Part model, mm, in its own coordinate system. A direction names the side the tool comes from. Round coordinates to 2 decimals unless told otherwise and drop trailing zeros. Write each loop counter-clockwise with the first axis right and the second up, starting at its lowest first coordinate (ties: lowest second). Pieces come first, ordered by that corner, then holes.
1) Drill centre lines: L1, parallel to Y at x = -35, z = 78; L2, parallel to X at y = 42, z = 18; L3, parallel to Z at x = -72.5, y = 26. Where is each one in solid material? Low to high.
2) Pull direction Z, two halves, no side cores. Call faces 1 (the flat face through (-22.76, -3.7, 105.18)), 2 (the flat face through (-81, -3, 0)), 3 (the flat face through (-28, -62.49, 40)), 4 (the flat face through (-26.974, -5.309, 113.826)): +Z half, -Z half, draft (parallel to the pull), parting line (faces both ways), or undercut.
3) Saw through at C-C on x = -71.5. Write the cut outline in (y, z), and give its area (3 significant figures).
4) Flat gauge pins, fed straight in: pin 1 (2 mm diameter, centred on x = -67, y = -57, fed in from -Z); pin 2 (2 mm diameter, centred on y = -2, z = 126, fed in from +X); pin 3 (1.5 mm diameter, centred on x = -33, y = 11.5, fed in from +Z). Where does each tip first touch, or does it go through?
5) Saw through at D-D on z = 86.5. Write the cut outline in (x, y), and give its area (3 significant figures).
6) Saw through at A-A on y = -22. Write the cut outline in (x, z) (3 decimals), and give its area (3 significant figures).
7) Which spindle directions (+Z, -Z, +X, -X, +Y, -Y) get a long thin tool onto all of the face, cutting with end or side? Do faces 5 (the flat face through (-79.493, -5, 52)), 6 (the flat face through (-51, -3, 105)), 7 (the flat face through (51.551, -5, 14)). Say none if no direction does.
8) Saw through at B-B on x = 34. Write the cut outline in (y, z).
```python
from build123d import *

# Parameters (mm, degrees)
SKETCH3_W           = 150
SKETCH3_H           = 150
BOSS_EXTRUDE2_DEPTH = 150
CUT_EXTRUDE3_DEPTH  = 150
SKETCH8_W           = 131.044313332
SKETCH8_H           = 116.977993985
CUT_EXTRUDE7_DEPTH  = 105
SKETCH9_W           = 4.954866237
SKETCH9_H           = 116.977993985
CUT_EXTRUDE10_DEPTH = 3
SKETCH10_W          = 105.341543671
SKETCH10_H          = 5
CUT_EXTRUDE12_DEPTH = 3
SKETCH11_W          = 5
SKETCH11_H          = 121.977993985
CUT_EXTRUDE13_DEPTH = 3
SKETCH12_W          = 110.341543671
SKETCH12_H          = 5
CUT_EXTRUDE14_DEPTH = 3


with BuildPart() as part:
    # Sketch3 → Boss-Extrude2 (new body)
    with BuildSketch(Plane.XY):
        with Locations((-13.712644514, -4.259252527)):
            Rectangle(SKETCH3_W, SKETCH3_H)
    extrude(amount=BOSS_EXTRUDE2_DEPTH)

    # Sketch6 → Cut-Extrude3 (cut)
    with BuildSketch(Plane.XZ.offset(79.259252527)):
        Polygon((61.287355486, 22.975304178), (-62.11733168, 150), (61.287355486, 150), align=None)
    extrude(amount=-CUT_EXTRUDE3_DEPTH, mode=Mode.SUBTRACT)

    # Sketch8 → Cut-Extrude7 (cut)
    with BuildSketch(Plane(origin=(0, 0, 0), x_dir=(-1, 0, 0), z_dir=(0, 0, -1))):
        with Locations((13.971216561, -4.00068048)):
            Rectangle(SKETCH8_W, SKETCH8_H)
    extrude(amount=-CUT_EXTRUDE7_DEPTH, mode=Mode.SUBTRACT)

    # Sketch9 → Cut-Extrude10 (cut)
    with BuildSketch(Plane(origin=(43.01226643, 0, 41.786482925), x_dir=(0.696812609304925, 0, -0.71725322412218), z_dir=(0.71725322412218, 0, 0.696812609304925))):
        with Locations((-90.610208196, -4.00068048)):
            Rectangle(SKETCH9_W, SKETCH9_H)
    extrude(amount=-CUT_EXTRUDE10_DEPTH, mode=Mode.SUBTRACT)

    # Sketch10 → Cut-Extrude12 (cut)
    with BuildSketch(Plane(origin=(43.01226643, 0, 41.786482925), x_dir=(0.696812609304925, 0, -0.71725322412218), z_dir=(0.71725322412218, 0, 0.696812609304925))):
        with Locations((-40.416869479, -64.989677472)):
            Rectangle(SKETCH10_W, SKETCH10_H)
    extrude(amount=-CUT_EXTRUDE12_DEPTH, mode=Mode.SUBTRACT)

    # Sketch11 → Cut-Extrude13 (cut)
    with BuildSketch(Plane(origin=(43.01226643, 0, 41.786482925), x_dir=(0.696812609304925, 0, -0.71725322412218), z_dir=(0.71725322412218, 0, 0.696812609304925))):
        with Locations((14.753902357, -6.50068048)):
            Rectangle(SKETCH11_W, SKETCH11_H)
    extrude(amount=-CUT_EXTRUDE13_DEPTH, mode=Mode.SUBTRACT)

    # Sketch12 → Cut-Extrude14 (cut)
    with BuildSketch(Plane(origin=(43.01226643, 0, 41.786482925), x_dir=(0.696812609304925, 0, -0.71725322412218), z_dir=(0.71725322412218, 0, 0.696812609304925))):
        with Locations((-37.916869479, 56.988316513)):
            Rectangle(SKETCH12_W, SKETCH12_H)
    extrude(amount=-CUT_EXTRUDE14_DEPTH, mode=Mode.SUBTRACT)


solid = part.part
```
Completed:
1. L1: y = -79.26 to -62.49, 54.49 to 70.74
1. L2: x = -88.71 to -79.49, 51.55 to 61.29
1. L3: z = 105 to 150
2. face 1: undercut
2. face 2: -Z half
2. face 3: draft
2. face 4: +Z half
3. outline: (-79.26, 0) - (-62.49, 0) - (-62.49, 105) - (54.49, 105) - (54.49, 0) - (70.74, 0) - (70.74, 150) - (-79.26, 150) - close
3. area: 10,200 mm2
4. pin 1: stops at z = 105
4. pin 2: stops at x = -37.83
4. pin 3: stops at z = 120.8
5. outline: (-88.71, -79.26) - (-0.43, -79.26) - (-0.43, -67.49) - (-4.61, -67.49) - (-4.61, -62.49) - (-79.49, -62.49) - (-79.49, 54.49) - (-4.61, 54.49) - (-4.61, 59.49) - (-0.43, 59.49) - (-0.43, 70.74) - (-88.71, 70.74) - close
5. area: 3,950 mm2
6. outline: (-88.713, 0) - (-79.493, 0) - (-79.493, 105) - (-22.582, 105) - (-24.004, 106.463) - (-21.852, 108.554) - (-62.117, 150) - (-88.713, 150) - close; (51.551, 0) - (61.287, 0) - (61.287, 22.975) - (55.035, 29.411) - (52.883, 27.321) - (51.551, 28.692) - close
6. area: 3,400 mm2
7. face 5: -Z
7. face 6: -Z, +X
7. face 7: +Z, -Z
8. outline: (-79.26, 0) - (-62.49, 0) - (-62.49, 46.76) - (-67.49, 46.76) - (-67.49, 51.06) - (-79.26, 51.06) - close; (54.49, 0) - (70.74, 0) - (70.74, 51.06) - (59.49, 51.06) - (59.49, 46.76) - (54.49, 46.76) - close
